Part model, mm, in its own coordinate system. A direction names the side the tool comes from. Coordinates: 2 decimals unless noted, no trailing zeros. Loops run counter-clockwise (first coordinate to the right, second up) from the corner with the lowest first, then second, coordinate; pieces in that order, holes last. Notation, with made-up numbers: M -14,-5.5 L 34,-5.5 A22 ccw 34,25.5 Z; hole C -8,-26.5 d4. An arc over 180 degrees is marked long. Use a Markdown table: item, result. Add a question column.
1) Band-saw the part on B-B (z = 0). List the corners of the cut face in (x, y), plus the area to 3 significant figures.
2) Tool access for faces 1 (the flat face through (4, 9, 0)), 2 (the flat face through (-12.4, -1, 7.3)), 3 (the flat face through (-7.229, 4, -6)): list every direction of +Z, -Z, +X, -X, +Y, -Y with a clear straight run to the whole face (end or side of a thin tool).
3) Band-saw the part on C-C (y = -7.25). List the corners of the cut face in (x, z), plus the area to 3 significant figures.
4) Pin check, flat tips, straight feed: pin 1 Ø1.5 at (x, z) = (-15, -6.5) entering from +Y; pin 2 Ø6.5 at (x, z) = (-10, 6) entering from +Y; pin 3 Ø5 at (x, y) = (-14.5, 5.5) entering from -Z; pin 4 Ø5 at (x, y) = (-14.5, 6) entering from +Z. Stop position of each tip, or through.
5) Band-saw the part on D-D (y = 7). List the corners of the cut face in (x, z), plus the area to 3 significant figures.
6) Band-saw the part on A-A (x = -12.5). List the corners of the cut face in (y, z).
7) Wall check: probe 1 along X at (y, z) = (-6, -5.5); probe 2 along X at (y, z) = (-3, -7.75); probe 3 along X at (y, z) = (4.75, -6.75). Give the ranges that are in metal, low to high. Write a range as from..to.
8) Pull direction Y, two halves, no side cores. Call faces 4 (the cylindrical face through (-22.4, -0.1, 2.5)), 5 (the flat face through (-12.4, -1, -7.4)), 6 (the flat face through (17.4, 4, 4)), 7 (the cylindrical face through (-13.92, -4.94, 6.24)): released by +Y, released by -Y, zero draft, split by the parting line, or undercut.
from build123d import *

# Parameters (mm, degrees)
SKETCH_1_W          = 35
SKETCH_1_H          = 18
EXTRUDE_1_DEPTH     = 9
SKETCH_2_R          = 6.015690921
SKETCH_2_R_2        = 5.389890323
CUT_EXTRUDE_1_DEPTH = 0.1
SKETCH_3_R          = 1.6
CUT_EXTRUDE_2_DEPTH = 27.669270706
SKETCH_4_R          = 2.5
EXTRUDE_2_DEPTH     = 10
SKETCH_5_W          = 10.271095748
SKETCH_5_H          = 5.975058515
CUT_EXTRUDE_3_DEPTH = 10


with BuildPart() as part:
    # 草图1 → 凸台-拉伸1 (new, symmetric)
    with BuildSketch(Plane(origin=(0, 0, 0), x_dir=(1, 0, 0), z_dir=(0, 1, 0))):
        Rectangle(SKETCH_1_W, SKETCH_1_H)
    extrude(amount=EXTRUDE_1_DEPTH, both=True)

    # 草图2 → 切除-拉伸1 (cut)
    with BuildSketch(Plane(origin=(17.5, 0, 0), x_dir=(0, 0, -1), z_dir=(1, 0, 0))):
        Circle(SKETCH_2_R)
        Circle(SKETCH_2_R_2, mode=Mode.SUBTRACT)
    extrude(amount=-CUT_EXTRUDE_1_DEPTH, mode=Mode.SUBTRACT)

    # 草图3 → 切除-拉伸2 (cut, through all)
    with BuildSketch(Plane(origin=(0, 9, 0), x_dir=(1, 0, 0), z_dir=(0, 1, 0))):
        with Locations(Location((-12.5, 5.5, 0), (0, 0, 270))):
            Circle(SKETCH_3_R)
        with Locations(Location((-12.5, -5.5, 0), (0, 0, 270))):
            Circle(SKETCH_3_R)
    extrude(amount=-CUT_EXTRUDE_2_DEPTH, mode=Mode.SUBTRACT)

    # 草图4 → 凸台-拉伸2 (add)
    with BuildSketch(Plane.ZY.offset(17.5)):
        with Locations(Location((0, 0, 0), (0, 0, 180))):
            Circle(SKETCH_4_R)
    extrude(amount=EXTRUDE_2_DEPTH)

    # 草图5 → 切除-拉伸3 (cut)
    with BuildSketch(Plane(origin=(0, 9, 0), x_dir=(1, 0, 0), z_dir=(0, 1, 0))):
        with Locations((-12.364452126, 6.012470742)):
            Rectangle(SKETCH_5_W, SKETCH_5_H)
        with Locations((-12.364452126, -6.012470742)):
            Rectangle(SKETCH_5_W, SKETCH_5_H)
    extrude(amount=-CUT_EXTRUDE_3_DEPTH, mode=Mode.SUBTRACT)


solid = part.part
Entries:
| question | item | result |
|---|---|---|
| 1 | outline | M -27.5,-2.5 L -17.5,-2.5 L -17.5,-9 L 17.5,-9 L 17.5,-6.02 L 17.4,-6.02 L 17.4,-5.39 L 17.5,-5.39 L 17.5,5.39 L 17.4,5.39 L 17.4,6.02 L 17.5,6.02 L 17.5,9 L -17.5,9 L -17.5,2.5 L -27.5,2.5 Z |
| 1 | area | 680 mm2 |
| 2 | face 1 | +Z, -Z, +X, -X, +Y |
| 2 | face 2 | +Z, -X, +Y |
| 2 | face 3 | -Z, -X, +Y |
| 3 | outline | M -17.5,-9 L 17.5,-9 L 17.5,9 L -17.5,9 Z; hole C -12.5,-5.5 d3.2; hole C -12.5,5.5 d3.2 |
| 3 | area | 614 mm2 |
| 4 | pin 1 | y = -1 |
| 4 | pin 2 | y = 9 |
| 4 | pin 3 | z = -3.02 |
| 4 | pin 4 | z = 3.02 |
| 5 | outline | M -17.5,-3.02 L -7.23,-3.02 L -7.23,-9 L 17.5,-9 L 17.5,9 L -7.23,9 L -7.23,3.02 L -17.5,3.02 Z |
| 5 | area | 507 mm2 |
| 6 | outline | M -9,-9 L -1,-9 L -1,-7.1 L -9,-7.1 Z; M -9,-3.9 L -1,-3.9 L -1,-3.02 L 9,-3.02 L 9,3.02 L -1,3.02 L -1,3.9 L -9,3.9 Z; M -9,7.1 L -1,7.1 L -1,9 L -9,9 Z |
| 7 | probe 1 | -17.5..-14.1, -10.9..17.5 |
| 7 | probe 2 | -17.5..17.5 |
| 7 | probe 3 | -7.23..17.5 |
| 8 | face 4 | split by the parting line |
| 8 | face 5 | released by +Y |
| 8 | face 6 | undercut |
| 8 | face 7 | zero draft |
